Model file for the job. Use its own axes, mm. Face numbers are marked on the shaded views. Round coordinates to 2 decimals unless told otherwise and drop trailing zeros. Order: outer loops, then holes, each group sorted by start corner. A loop starts at its lowest first (then second) coordinate and runs counter-clockwise, first axis right, second up. Notation, with made-up numbers: (71, 3.5) - (79, 3.5) arc R14 cw to (79, 26.5) - close; hole circle Ø6 at (-19, 71). An arc over 180 degrees is marked (long way). Put each result on its own line as item: value. Start each with the question number.
Item 1: Saw through at A-A on y = -11. List the corners of the cut face in (x, z), plus the area to 3 significant figures.
Item 2: Probe probe 1 along Y at (x, z) = (-48.25, 2); probe 2 along Y at (x, z) = (46, -0.95); probe 3 along Z at (x, y) = (15, -4.5). List the from-to ranges inside material, lowest first.
Item 3: Saw through at B-B on z = -0.75. State how many separate pieces and enclosed holes the cut face has, plus the area to 3 significant figures.
Item 4: Saw through at C-C on x = 13. List the corners of the cut face in (y, z), plus the area to 3 significant figures.
Item 5: Mould opens along X. For the marked faces 1 and 2 say: pulls with the +X half, pulls with the -X half, needs draft (parallel to the pull), parting line crosses it, or undercut.
Item 6: Pin check, flat tips, straight feed: pin 1 Ø1.9 at (x, y) = (48.25, -58.436) entering from +Z; pin 2 Ø1.5 at (x, y) = (11, 15.5) entering from -Z; pin 3 Ø4 at (x, y) = (48.25, 58.436) entering from +Z. Stop position of each tip, or through.
```python
from build123d import *

# Parameters (mm, degrees)
SKETCH_W        = 116.5
SKETCH_H        = 165
PAD_DEPTH       = 3
PAD001_DEPTH    = 165
SKETCH002_R     = 1.6
POCKET_DEPTH    = 4.5
SKETCH003_W     = 9.5
SKETCH003_H     = 9.5
POCKET001_DEPTH = 1.5
FILLET_R        = 5


with BuildPart() as part:
    # Sketch → Pad (new body)
    with BuildSketch(Plane.XY):
        Rectangle(SKETCH_W, SKETCH_H)
    extrude(amount=PAD_DEPTH)

    # Sketch001 (on Face3 of Pad) → Pad001 (join)
    with BuildSketch(Plane.XZ.offset(82.5)):
        Polygon((-53, 0), (-43.5, 0), (-45.3, -1.5), (-51.2, -1.5), align=None)
    pad001 = extrude(amount=-PAD001_DEPTH)

    # Sketch002 (on Face10 of Pad001) → Pocket (cut)
    with BuildSketch(Plane(origin=(0, 0, -1.5), x_dir=(1, 0, 0), z_dir=(0, 0, -1))):
        with Locations((-48.25, -24.064)):
            Circle(SKETCH002_R)
        with Locations((-48.25, -58.436)):
            Circle(SKETCH002_R)
        with Locations((-48.25, 58.436)):
            Circle(SKETCH002_R)
        with Locations((-48.25, 24.064)):
            Circle(SKETCH002_R)
    pocket = extrude(amount=-POCKET_DEPTH, mode=Mode.SUBTRACT)

    # Sketch003 (on Face10 of Pocket) → Pocket001 (cut)
    with BuildSketch(Plane(origin=(0, 0, -1.5), x_dir=(1, 0, 0), z_dir=(0, 0, -1))):
        with Locations((-48.25, 24.064)):
            Rectangle(SKETCH003_W, SKETCH003_H)
        with Locations((-48.25, 58.436)):
            Rectangle(SKETCH003_W, SKETCH003_H)
        with Locations((-48.25, -24.064)):
            Rectangle(SKETCH003_W, SKETCH003_H)
        with Locations((-48.25, -58.436)):
            Rectangle(SKETCH003_W, SKETCH003_H)
    pocket001 = extrude(amount=-POCKET001_DEPTH, mode=Mode.SUBTRACT)

    # Mirrored: Pad001, Pocket, Pocket001 across YZ
    add(pad001.mirror(Plane.YZ))
    add(pocket.mirror(Plane.YZ), mode=Mode.SUBTRACT)
    add(pocket001.mirror(Plane.YZ), mode=Mode.SUBTRACT)

    # Fillet
    fillet_edges = [part.edges().sort_by_distance(p)[0] for p in [
        (58.25, 82.5, 1.5),
        (-58.25, 82.5, 1.5),
        (58.25, -82.5, 1.5),
        (-58.25, -82.5, 1.5),
    ]]
    fillet(fillet_edges, radius=FILLET_R)


solid = part.part
```
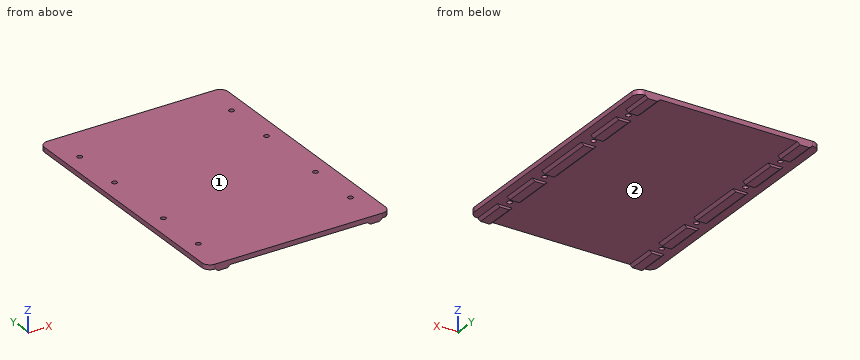
Results found:
1. outline: (-58.25, 0) - (-53, 0) - (-51.2, -1.5) - (-45.3, -1.5) - (-43.5, 0) - (43.5, 0) - (45.3, -1.5) - (51.2, -1.5) - (53, 0) - (58.25, 0) - (58.25, 3) - (-58.25, 3) - close
1. area: 373 mm²
2. probe 1: y = -82.5 to -60.04, -56.84 to -25.66, -22.46 to 22.46, 25.66 to 56.84, 60.04 to 82.5
2. probe 2: y = -82.5 to -63.19, -53.69 to -28.81, -19.31 to 19.31, 28.81 to 53.69, 63.19 to 82.5
2. probe 3: z = 0 to 3
3. separate pieces: 10
3. enclosed holes: 0
3. area: 1,960 mm²
4. outline: (-82.5, 0) - (82.5, 0) - (82.5, 3) - (-82.5, 3) - close
4. area: 495 mm²
5. face 1: needs draft
5. face 2: undercut
6. pin 1: passes through
6. pin 2: stops at z = 0
6. pin 3: stops at z = 3
